For this review, take the finished solid that the model builds, in its own axes (mm). A direction names the side the tool comes from. Give positions to 0.01 mm unless a question says otherwise; leave off trailing zeros. Order: outer loops, then holes, each group sorted by start corner. A loop starts at its lowest first (then second) coordinate and runs counter-clockwise, first axis right, second up.
from build123d import *

# Parameters (mm, degrees)
SKETCH1_R      = 0.9
EXTRUDE1_DEPTH = 3


with BuildPart() as part:
    # Sketch1 → Extrude1 (new body)
    with BuildSketch(Plane(origin=(0, 0, 0), x_dir=(0, 0, -1), z_dir=(1, 0, 0))):
        with BuildLine():
            Line((0, 0), (23, 0))
            ThreePointArc((23, 0), (25.882785208, 4.750682993), (20.337755856, 5.114123418))
            Line((20.337755856, 5.114123418), (19.55763824, 4))
            Line((19.55763824, 4), (0, 4))
            ThreePointArc((0, 4), (-2, 2), (0, 0))
        make_face()
        with Locations((0, 2)):
            Circle(SKETCH1_R, mode=Mode.SUBTRACT)
        with BuildLine():
            Line((24.1, 4.15), (24.1, 2.35))
            ThreePointArc((24.1, 2.35), (23, 1.25), (21.9, 2.35))
            Line((21.9, 2.35), (21.9, 4.15))
            ThreePointArc((21.9, 4.15), (23, 5.25), (24.1, 4.15))
        make_face(mode=Mode.SUBTRACT)
    extrude(amount=EXTRUDE1_DEPTH)


solid = part.part
1) Clearance check with flat-ended pins moving along their axes: pin 1 (1.5 mm diameter, centred on x = 2.5, y = 4, fed in from -Z); pin 2 (1.5 mm diameter, centred on x = 2.5, y = 5.5, fed in from -Z); pin 3 (1 mm diameter, centred on x = 0.5, z = -12, fed in from +Y); pin 4 (0.5 mm diameter, centred on x = 1.5, y = 3.5, fed in from +Z). State where each tip first meets the part, or that it passes through.
Answer sheet:
pin 1: stops at z = -26.25
pin 2: stops at z = -25.88
pin 3: stops at y = 4
pin 4: stops at z = 1.56
2) Tool access review of faces 1 (the face through (3, 2, -15)), 2 (the face through (1, 4, -10)), 3 (the face through (1, 3, -21.9)): name each direction out of +Z, -Z, +X, -X, +Y, -Y from which nothing blocks a thin tool from reaching the whole face with its end or side.
Answer sheet:
face 1: +Z, -Z, +X, +Y, -Y
face 2: +Z, +X, -X, +Y
face 3: +X, -X
3) We need section A-A on y = 4.5. Give the boundary of the cut face in (x, z), then the cut area to 3 significant figures.
Answer sheet:
outline: (0, -26) - (3, -26) - (3, -24.04) - (0, -24.04) - close; (0, -21.96) - (3, -21.96) - (3, -19.91) - (0, -19.91) - close
area: 12.0 mm2
4) To check wall thickness, follow line 1 (Z direction, x = 0.8, y = 2.5); line 2 (Z direction, x = 0.85, y = 2.75); line 3 (Y direction, x = 0.35, z = -1). State the ranges of each line that lie inside material, in increasing order.
Answer sheet:
line 1: z = -26.16 to -24.1, -21.9 to -0.75, 0.75 to 1.94
line 2: z = -26.21 to -24.1, -21.9 to -0.5, 0.5 to 1.85
line 3: y = 0 to 4
5) We need section B-B on x = 0.8. Give the boundary of the cut face in (y, z), then the cut area to 3 significant figures.
Answer sheet:
outline: (0, -23) arc R3.25 ccw (long way) to (5.11, -20.34) - (4, -19.56) - (4, 0) arc R2 ccw to (0, 0) - close; hole circle Ø1.8 at (2, 0); hole (2.35, -24.1) - (4.15, -24.1) arc R1.1 ccw to (4.15, -21.9) - (2.35, -21.9) arc R1.1 ccw to start
area: 111 mm2
6) We need section D-D on z = -8.75. Give the boundary of the cut face in (x, y).
Answer sheet:
outline: (0, 0) - (3, 0) - (3, 4) - (0, 4) - close
7) We need section C-C on y = 2. Give the boundary of the cut face in (x, z).
Answer sheet:
outline: (0, -26) - (3, -26) - (3, -24.04) - (0, -24.04) - close; (0, -21.96) - (3, -21.96) - (3, -0.9) - (0, -0.9) - close; (0, 0.9) - (3, 0.9) - (3, 2) - (0, 2) - close
8) Draft analysis for pull direction Z (two halves, no side actions). For faces 4 (the face through (0, 2, -15)), 5 (the face through (1.48, 5.25, -22.98)), 6 (the face through (1.48, 4.56, -19.95)), state which applies: +Z half, -Z half, draft (parallel to the pull), parting line (faces both ways), or undercut.
Answer sheet:
face 4: draft
face 5: undercut
face 6: +Z half
